from build123d import *

# Parameters (mm, degrees)
SKETCH1_R             = 2.5
BOSS_EXTRUDE1_DEPTH   = 2.5
BOSS_EXTRUDE1_2_DEPTH = 2.5
SKETCH2_R             = 4
SKETCH2_R_2           = 2.5
BOSS_EXTRUDE2_DEPTH   = 0.5
SKETCH3_R             = 1
CUT_EXTRUDE1_DEPTH    = 12.497479072


with BuildPart() as part:
    # Sketch1 → Boss-Extrude1 (new, symmetric)
    with BuildSketch(Plane.YZ):
        with Locations(Location((-4.955, 0, 0), (0, 0, 270))):
            Circle(SKETCH1_R)
    extrude(amount=BOSS_EXTRUDE1_DEPTH, both=True)



with BuildPart() as body_2:
    # Sketch1 → Boss-Extrude1 2 (new, symmetric)
    with BuildSketch(Plane.YZ):
        with Locations(Location((4.955, 0, 0), (0, 0, 90))):
            Circle(SKETCH1_R)
    extrude(amount=BOSS_EXTRUDE1_2_DEPTH, both=True)


with BuildPart() as part_1:
    add(part.part)

    add(body_2.part)  # Boss-Extrude2 merges body 2
    # Sketch2 → Boss-Extrude2 (add, symmetric)
    # profile 1 of 4: a face of its own
    with BuildSketch(Plane.YZ.offset(2.5)):
        with Locations((-4.955, 0)):
            Circle(SKETCH2_R)
    # profile 2 of 4: a face of its own
    with BuildSketch(Plane.YZ.offset(2.5)):
        with BuildLine():
            ThreePointArc((-3.539285714, 3.741089823), (-1.663886424, 2.273449236), (-0.955, 0))
            ThreePointArc((-0.955, 0), (-1.663886424, -2.273449236), (-3.539285714, -3.741089823))
            ThreePointArc((-3.539285714, -3.741089823), (0, -3.093814379), (3.539285714, -3.741089823))
            ThreePointArc((3.539285714, -3.741089823), (0.955, 0), (3.539285714, 3.741089823))
            ThreePointArc((3.539285714, 3.741089823), (0, 3.093814379), (-3.539285714, 3.741089823))
        make_face()
    # profile 3 of 4: a face of its own
    with BuildSketch(Plane.YZ.offset(2.5)):
        with Locations((4.955, 0)):
            Circle(SKETCH2_R)
        with Locations(Location((4.955, 0, 0), (0, 0, 90))):
            Circle(SKETCH2_R_2, mode=Mode.SUBTRACT)
    # profile 4 of 4: a face of its own
    with BuildSketch(Plane.YZ.offset(2.5)):
        with Locations(Location((4.955, 0, 0), (0, 0, 90))):
            Circle(SKETCH2_R_2)
    boss_extrude2 = extrude(amount=BOSS_EXTRUDE2_DEPTH, both=True)

    # Mirror1: Boss-Extrude2 across plane
    add(boss_extrude2.mirror(Plane(origin=(0, 0, 0), x_dir=(0, 0, 1), z_dir=(1, 0, 0))))

    # Sketch3 → Cut-Extrude1 (cut, through all)
    with BuildSketch(Plane.YZ.offset(3)):
        with Locations(Location((-4.955, 0, 0), (0, 0, 270))):
            Circle(SKETCH3_R)
        with Locations(Location((4.955, 0, 0), (0, 0, 270))):
            Circle(SKETCH3_R)
    extrude(amount=-CUT_EXTRUDE1_DEPTH, mode=Mode.SUBTRACT)


solid = part_1.part
Read the model definition and answer for the solid it produces. Units are mm, in the model's axes. A direction names the side the tool comes from. Give positions to 0.01 mm unless a question says otherwise; leave off trailing zeros. Write each loop counter-clockwise with the first axis right and the second up, starting at its lowest first coordinate (ties: lowest second). Pieces come first, ordered by that corner, then holes. Notation, with made-up numbers: (45.25, 43.25) - (75.25, 43.25) arc R22 ccw to (75.25, 69.25) - close; hole circle Ø10 at (24.25, 41.5). An arc over 180 degrees is marked (long way). Answer in a Markdown table with one row per item. Add a question column.
Item 1: Section A-A, the plane z = 0 is taken. Write down the section's boundary in (x, y) (3 decimals), and give its area (3 significant figures).
Item 2: Section D-D, the plane z = -2 is taken. Write down the section's boundary in (x, y) (3 decimals).
Item 3: Section B-B, the plane y = -0.75 is taken. Write down the section's boundary in (x, z).
Item 4: Section C-C, the plane z = 3.5 is taken. Write down the section's boundary in (x, y).
Item 5: A tool of negligible diameter and unlimited length cuts with its end or side. For faces 1 (the face through (2, 0, 0)), 2 (the face through (-3, 0, 0)), from which of +Z, -Z, +X, -X, +Y, -Y can it reach the whole face along a straight path? Write none if from no direction.
Item 6: A flat-ended cylindrical pin translates along its axis: P1, Ø2, axis at x = -0.5, y = 4, coming from the +Z side. Find the tip coordinate at first contact, or state that the pin passes through.
Item 7: Find the intervals of material crossed by L1, parallel to Y at x = -1.15, z = 0 (3 decimals); L2, parallel to X at y = 1.75, z = 0.5; L3, parallel to Z at x = 0.9, y = 5, in increasing order.
Item 8: Determine the mould class of faces 3 (the face through (0.028, -2.847, -1.344)), 4 (the face through (3, 0, 0)) for opening direction Y: pulls with the +Y half, pulls with the -Y half, needs draft (parallel to the pull), parting line crosses it, or undercut.
Recorded:
| question | item | result |
|---|---|---|
| 1 | outline | (-3, -8.955) - (-2, -8.955) - (-2, -7.455) - (2, -7.455) - (2, -8.955) - (3, -8.955) - (3, -5.955) - (-3, -5.955) - close; (-3, -3.955) - (3, -3.955) - (3, 3.955) - (-3, 3.955) - close; (-3, 5.955) - (3, 5.955) - (3, 8.955) - (2, 8.955) - (2, 7.455) - (-2, 7.455) - (-2, 8.955) - (-3, 8.955) - close; hole (-2, -2.455) - (2, -2.455) - (2, 2.455) - (-2, 2.455) - close |
| 1 | area | 51.8 mm2 |
| 2 | outline | (-3, -8.419) - (-2, -8.419) - (-2, -6.455) - (2, -6.455) - (2, -8.419) - (3, -8.419) - (3, 8.419) - (2, 8.419) - (2, 6.455) - (-2, 6.455) - (-2, 8.419) - (-3, 8.419) - close; hole (-2, -3.455) - (2, -3.455) - (2, 3.455) - (-2, 3.455) - close |
| 3 | outline | (-3, -3.12) - (-2, -3.12) - (-2, 3.12) - (-3, 3.12) - close; (2, -3.12) - (3, -3.12) - (3, 3.12) - (2, 3.12) - close |
| 4 | outline | (-3, -6.89) - (-2, -6.89) - (-2, -2.82) - (-3, -2.82) - close; (-3, 2.82) - (-2, 2.82) - (-2, 6.89) - (-3, 6.89) - close; (2, -6.89) - (3, -6.89) - (3, -2.82) - (2, -2.82) - close; (2, 2.82) - (3, 2.82) - (3, 6.89) - (2, 6.89) - close |
| 5 | face 1 | none |
| 5 | face 2 | +Z, -Z, -X, +Y, -Y |
| 6 | P1 | stops at z = 2.5 |
| 7 | L1 | y = -7.455 to -5.955, -3.955 to -2.455, 2.455 to 3.955, 5.955 to 7.455 |
| 7 | L2 | x = -3 to -2, 2 to 3 |
| 7 | L3 | z = -2.5 to -1, 1 to 2.5 |
| 8 | face 3 | undercut |
| 8 | face 4 | needs draft |
